Autodesk Inventor part; units mm, degrees
ref_plane "YZ Plane" through (0, 0, 0) normal (1, 0, 0) x (0, 1, 0)
ref_plane "XZ Plane" through (0, 0, 0) normal (0, 1, 0) x (-1, 0, 0)
ref_plane "XY Plane" through (0, 0, 0) normal (0, 0, 1) x (1, 0, 0)
ref_plane "Work Plane1" through (-1.6596, -28.9901, 28.1919) normal (0, 0, 1) x (1, 0, 0)
sketch "Sketch1" plane through (-1.6596, -28.9901, 28.1919) normal (0, 0, 1) x (1, 0, 0)
  spline S0 degree 3 poles (-18.1261, -96.0287) (-18.1261, -96.0287) (-18.0932, -96.0287) (-18.0298, -96.0287) (-17.8251, -96.0287) (-17.2794, -96.0287) (-16.7467, -96.0287) (-16.213, -96.0287) (-15.7353, -96.0287) (-15.6244, -96.0287) (-15.6063, -96.0287) (-15.5971, -96.0287) (-15.5971, -96.0287) knots 0.499993 0.499993 0.499993 0.499993 0.562494 0.562494 0.562494 0.764477 0.764477 0.764477 0.966846 0.966846 0.966846 1 1 1 1 construction
  line L0 (-18.3185, -96.0287) -> (-15.9665, -96.0287) construction
  arc A0 (-13.8616, 2.5089) -> (-19.8616, 2.5089) centre (-16.8616, 2.5089) ccw construction
  arc A1 (-13.9993, -31.5037) -> (-19.9993, -31.5037) centre (-16.9993, -31.5037) ccw construction
  arc A2 (3.0015, -1.5044) -> (9.0015, -1.5044) centre (6.0015, -1.5044) ccw
  circle A3 centre (-16.8616, -31.5037) radius 1.6
  circle A4 centre (5.3371, -31.5037) radius 1.6
  circle A5 centre (-16.8616, 2.5089) radius 1.6
  circle A6 centre (5.3371, 2.5089) radius 1.6
  line L1 (-19.8616, 2.5089) -> (-22.8616, 2.5089) construction
  line L2 (6.9371, 2.5089) -> (11.3371, 2.5089) construction
  line L3 (-16.8616, -33.1037) -> (-16.8616, -36.2364) construction
  line L4 (-12.7018, 32.5036) -> (-22.8616, 2.5089)
  line L5 (-22.8616, 2.5089) -> (-22.8616, -36.2364)
  line L6 (7.9619, 32.5036) -> (11.3371, 2.5089)
  line L7 (11.3371, 2.5089) -> (11.3371, -36.2364)
  line L8 (11.3371, -36.2364) -> (-22.8616, -36.2364)
  line L9 (2.3051, 26.8467) -> (7.9619, 32.5036) construction
  line L10 (-12.7018, 32.5036) -> (7.9619, 32.5036)
  line L11 (2.3051, 26.8467) -> (-7.6949, 26.8467) construction
  line L12 (-19.8616, 78.2844) -> (-2.5116, 78.2844) construction
  line L13 (-11.1866, 78.2844) -> (-4.9166, 78.2844) construction
  line L14 (-11.1866, 78.2844) -> (-17.4566, 78.2844) construction
  line L15 (-19.8616, 78.2844) -> (-17.4566, 78.2844) construction
  line L16 (-4.9166, 78.2844) -> (-2.5116, 78.2844) construction
  line L17 (-7.6949, 26.8467) -> (-7.6949, 11.8467) construction
  circle A7 centre (-7.6949, 26.8467) radius 1.6
  circle A8 centre (-7.6949, 11.8467) radius 1.6
  line L18 (-7.6949, 11.8467) -> (2.3051, 11.8467) construction
  circle A9 centre (2.3051, 11.8467) radius 1.6
  circle A10 centre (2.3051, 26.8467) radius 1.6
  point P0 (1.6596, 28.9901)
  point P1 (-18.3185, 3.0171)
  point P2 (-15.9662, 3.4042)
  dimension "d5" = 3.2
  dimension "d8" = 3.2
  dimension "d6" = 3.2
  dimension "d7" = 3.2
  dimension "d51" = 3
  dimension "d52" = 4.4
  dimension "d56" = 8
  dimension "d58" = 10
  dimension "d59" = 17.35
  dimension "d60" = 6.27
  dimension "d61" = 6.27
  dimension "d62" = 15
  dimension "d63" = 3.2
  dimension "d64" = 3.2
  dimension "d65" = 3.2
  dimension "d66" = 3.2
ref_plane "Work Plane2" through (-8.6352, -23.8919, -35.0523) normal (0, 0, 1) x (1, 0, 0)
sketch "Sketch2" plane through (-8.6352, -23.8919, -35.0523) normal (0, 0, 1) x (1, 0, 0)
  line L0 (-7.5414, 41.3535) -> (-20.5414, 41.3535)
  line L1 (-20.5414, 44.5535) -> (-7.5414, 44.5535)
  line L2 (-7.5414, 44.5535) -> (-7.5414, 41.3535)
  line L3 (-20.5414, 41.3535) -> (-20.5414, 44.5535)
  line L4 (13.5, 41.3535) -> (0.5, 41.3535)
  line L5 (0.5, 44.5535) -> (13.5, 44.5535)
  line L6 (13.5, 44.5535) -> (13.5, 41.3535)
  line L7 (0.5, 41.3535) -> (0.5, 44.5535)
  line L8 (34.55, 41.3535) -> (21.55, 41.3535)
  line L9 (21.55, 44.5535) -> (34.55, 44.5535)
  line L10 (21.55, 41.3535) -> (21.55, 44.5535)
  line L11 (34.55, 44.5535) -> (34.55, 41.3535)
  line L12 (-14.0414, 44.5535) -> (-14.0414, 41.3535) construction
  line L13 (28.05, 44.5535) -> (28.05, 41.3535) construction
  circle A0 centre (-14.0414, 42.9535) radius 1.6
  circle A1 centre (28.05, 42.9535) radius 1.6
  point P0 (8.6352, 23.8919)
extrude "Extrusion1" add sketch "Sketch1" against normal blind 4.5
sketch "Sketch3" plane through (-1.6596, -28.9901, 28.1919) normal (0, 0, 1) x (1, 0, 0)
  line L0 (19.4071, -58.7998) -> (21.4071, -58.7998) construction
  line L1 (20.4071, -58.7998) -> (20.4979, -36.9098) construction
  line L2 (20.4979, -36.9098) -> (25.7879, -36.9098) construction
  line L3 (25.7879, -36.9098) -> (15.2079, -36.9098) construction
  circle A0 centre (15.2079, -36.9098) radius 1.6
  circle A1 centre (25.7879, -36.9098) radius 1.6
  circle A2 centre (15.2079, -36.9098) radius 4.6
  circle A3 centre (25.7879, -36.9098) radius 4.6
  line L4 (25.7879, -32.3098) -> (9.0007, -32.3098)
  line L5 (9.0007, -34.5533) -> (9.0007, 32.4467)
  line L6 (25.7879, -41.5098) -> (15.2079, -41.5098)
  line L7 (15.2079, -41.5098) -> (-19.9993, -41.5098)
  line L8 (-19.9993, -34.5533) -> (-19.9993, 32.4467)
  line L9 (-19.9993, -41.5098) -> (-19.9993, -34.5533)
  line L10 (-19.9993, -34.5533) -> (9.0007, -34.5533)
  line L11 (9.0007, -34.5533) -> (9.0007, -32.3098)
  line L12 (25.7879, -36.9098) -> (30.1497, -38.3706)
  line L13 (45.9071, 7.0963) -> (8.7371, 7.0963) construction
  line L14 (8.7371, 7.0963) -> (14.7371, 7.0963) construction
  line L15 (14.7371, 7.0963) -> (14.7371, -0.9037) construction
  line L16 (14.7371, -0.9037) -> (34.7371, -0.9037) construction
  line L17 (14.7371, -0.9037) -> (20.7371, -0.9037) construction
  line L18 (14.7371, -2.4037) -> (20.7371, -2.4037)
  line L19 (20.7371, 0.5963) -> (14.7371, 0.5963)
  arc A4 (14.7371, 0.5963) -> (14.7371, -2.4037) centre (14.7371, -0.9037) ccw
  arc A5 (20.7371, -2.4037) -> (20.7371, 0.5963) centre (20.7371, -0.9037) ccw
  line L20 (34.7371, -0.9037) -> (28.7371, -0.9037) construction
  line L21 (34.7371, 0.5963) -> (28.7371, 0.5963)
  line L22 (28.7371, -2.4037) -> (34.7371, -2.4037)
  arc A6 (34.7371, -2.4037) -> (34.7371, 0.5963) centre (34.7371, -0.9037) ccw
  arc A7 (28.7371, 0.5963) -> (28.7371, -2.4037) centre (28.7371, -0.9037) ccw
  line L23 (34.7371, 3.5963) -> (28.7371, 3.5963)
  arc A8 (28.7371, 3.5963) -> (28.7371, -5.4037) centre (28.7371, -0.9037) ccw
  line L24 (28.7371, -5.4037) -> (34.7371, -5.4037)
  arc A9 (34.7371, -5.4037) -> (34.7371, 3.5963) centre (34.7371, -0.9037) ccw
  line L25 (28.7371, 3.5963) -> (9.0007, 3.5963)
  line L26 (28.7371, -5.4037) -> (9.0007, -5.4037)
  line L27 (11.3371, -36.2364) -> (-22.8616, -36.2364)
  line L28 (-22.8616, -36.2364) -> (-22.8616, -41.5098)
  line L29 (-22.8616, -41.5098) -> (-19.9993, -41.5098)
  point P0 (1.6596, 28.9901)
  point P1 (11.4479, -23.0098)
  point P2 (9.0007, -15.5098)
  point P3 (17.7371, -0.9037)
  point P4 (31.7371, -0.9037)
  point P5 (-19.9993, -36.2364)
  dimension "d9" = 10.58
  dimension "d10" = 5.29
  dimension "d11" = 10.58
  dimension "d12" = 3.2
  dimension "d13" = 3.2
  dimension "d14" = 3
  dimension "d15" = 3
  dimension "d43" = 6
  dimension "d44" = 8
  dimension "d45" = 20
  dimension "d46" = 6
  dimension "d47" = 3
  dimension "d48" = 6
  dimension "d49" = 3
  dimension "d50" = 3
extrude "Extrusion2" add sketch "Sketch3" against normal blind 4.5
sketch "Sketch4" plane through (-1.6596, -28.9901, 23.6919) normal (0, 0, -1) x (-1, 0, 0)
  circle A0 centre (-2.3051, 26.8467) radius 1.6
  circle A1 centre (-2.3051, 26.8467) radius 3
  circle A2 centre (7.6949, 26.8467) radius 1.6
  circle A3 centre (7.6949, 26.8467) radius 3
  circle A4 centre (7.6949, 11.8467) radius 1.6
  circle A5 centre (7.6949, 11.8467) radius 3
  circle A6 centre (-2.3051, 11.8467) radius 1.6
  circle A7 centre (-2.3051, 11.8467) radius 3
  dimension "d67" = 6
  dimension "d68" = 6
  dimension "d69" = 6
  dimension "d70" = 6
extrude "Extrusion3" cut sketch "Sketch4" against normal blind 3.5
fillet "Fillet1" radius 2 7 edges at (-24.5212, -70.4999, 25.9419) (9.6775, -34.3938, 25.9419) (9.6775, -61.2999, 25.9419) (9.5552, -25.3938, 25.9419) (-14.3614, 3.5135, 25.9419) (6.3023, 3.5135, 25.9419) (-24.5212, -26.4812, 25.9419)
sketch "Sketch5" plane through (-1.6596, -28.9901, 28.1919) normal (0, 0, 1) x (1, 0, 0)
  circle A0 centre (-16.8616, 2.5089) radius 1.6
  circle A1 centre (-16.8616, 2.5089) radius 3
  circle A2 centre (5.3371, 2.5089) radius 1.6
  circle A3 centre (5.3371, 2.5089) radius 3
  circle A4 centre (-16.8616, -31.5037) radius 1.6
  circle A5 centre (-16.8616, -31.5037) radius 3
  circle A6 centre (5.3371, -31.5037) radius 1.6
  circle A7 centre (5.3371, -31.5037) radius 3
  point P0 (1.6596, 28.9901)
  dimension "d25" = 6
  dimension "d26" = 6
  dimension "d27" = 6
  dimension "d28" = 6
extrude "Extrusion4" cut sketch "Sketch5" against normal blind 3.5 contours A1 | A2 | A3 | A5 | A7
properties part number "rails-bolts"
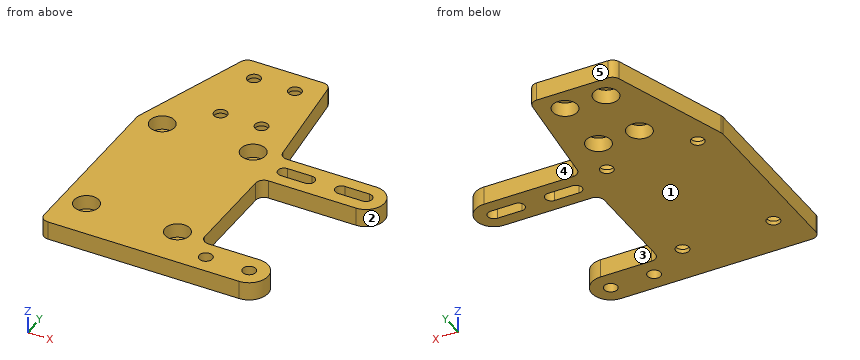
For this review, take the finished solid that the model builds, in its own axes (mm). Face numbers are marked on the shaded views. A direction names the side the tool comes from. Coordinates: 2 decimals unless noted, no trailing zeros. Order: outer loops, then holes, each group sorted by start corner. A loop starts at its lowest first (then second) coordinate and runs counter-clockwise, first axis right, second up. Notation, with made-up numbers: (38, 3) - (59, 3) arc R11 ccw to (59, 24) - close; hole circle Ø9 at (11, 24.25). An arc over 180 degrees is marked (long way). Answer as a JSON object with one key per item and string values. Group by question number.
1. For the marked faces 4 and 5, list the 3-axis set-ups (+Z, -Z, +X, -X, +Y, -Y) from which the entire face can be reached by the end or side of a thin tool; tool diameter is ignored.
2. We need section D-D on z = 26.25. Give the number of separate pieces and of enclosed holes in the cut face, then the cut area to 3 significant figures.
3. We need section B-B on x = 32. State the section outline as (y, z) points.
4. Clearance check with flat-ended pins moving along their axes: P1, Ø3.5, axis at x = 13.55, y = -65.9, coming from the -Z side; P2, Ø5, axis at x = 3.68, y = -60.49, coming from the +Z side; P3, Ø2, axis at x = 22, z = 25, coming from the +Y side; P4, Ø1.8, axis at x = -9, y = -3, coming from the -Z side. State where each tip first meets the part, or that it passes through.
5. We need section C-C on y = -54. State the section outline as (x, z) points, then the cut area to 3 significant figures.
6. For probe 1 along X at (y, z) = (-66, 27.45); probe 2 along Y at (x, z) = (14, 24.8); probe 3 along X at (y, z) = (-3.5, 27.05), list the stretches that pass through material, from the lowest coordinate up.
7. We need section A-A on x = 21.5. State the section outline as (y, z) points, then the cut area to 3 significant figures.
8. The part is to be moulded in two halves that separate along Y. For the marked faces 1, 2 and 3, say which applies: pulls with the +Y half, pulls with the -Y half, needs draft (parallel to the pull), parting line crosses it, or undercut.
Final values:
{
 "1": {"face 4": "+Z, -Z, +X, +Y", "face 5": "+Z, -Z, +X, -X, +Y"},
 "2": {"separate pieces": "1", "enclosed holes": "12", "area": "2,440 mm²"},
 "3": {"outline": "(-34.39, 23.69) - (-31.39, 23.69) - (-31.39, 28.19) - (-34.39, 28.19) - close; (-28.39, 23.69) - (-25.39, 23.69) - (-25.39, 28.19) - (-28.39, 28.19) - close"},
 "4": {"P1": "z = 23.69", "P2": "z = 24.69", "P3": "y = -25.39", "P4": "z = 27.19"},
 "5": {"outline": "(-24.52, 23.69) - (9.68, 23.69) - (9.68, 28.19) - (-24.52, 28.19) - close", "area": "154 mm²"},
 "6": {"probe 1": "-24.52 to 11.95, 15.15 to 22.53, 25.73 to 28.73", "probe 2": "-70.5 to -67.43, -64.36 to -61.3, -34.39 to -31.39, -28.39 to -25.39", "probe 3": "-16.74 to -12.03, -6.68 to -2.03, 3.32 to 7.09"},
 "7": {"outline": "(-70.5, 23.69) - (-61.3, 23.69) - (-61.3, 28.19) - (-70.5, 28.19) - close; (-34.39, 23.69) - (-25.39, 23.69) - (-25.39, 28.19) - (-34.39, 28.19) - close", "area": "81.9 mm²"},
 "8": {"face 1": "needs draft", "face 2": "parting line crosses it", "face 3": "undercut"}
}
